Here's how the part is built. I have some questions about the finished solid (model axes, mm). Round coordinates to 2 decimals unless told otherwise and drop trailing zeros. Write each loop counter-clockwise with the first axis right and the second up, starting at its lowest first coordinate (ties: lowest second). Pieces come first, ordered by that corner, then holes. Notation, with made-up numbers: M 9,59.25 L 54,59.25 A19 cw 54,81.25 Z; hole C 63.25,-28 d7. An arc over 180 degrees is marked long. Use a Markdown table: item, result. Add a question column.
```python
from build123d import *

# Parameters (mm, degrees)
BOSS_EXTRUDE1_DEPTH = 152.4
SKETCH3_OUTSIDE_W   = 237.922
SKETCH3_OUTSIDE_H   = 226.36
CUT_EXTRUDE2_DEPTH  = 365.792952335
SHELL1_T            = -6.35
SKETCH8_W           = 266.062607669
SKETCH8_H           = 282.191647152
CUT_EXTRUDE6_DEPTH  = 300.618382774
CUT_EXTRUDE3_DEPTH  = 350.742043935
SKETCH5_OUTSIDE_W   = 351.444
SKETCH5_OUTSIDE_H   = 196.758
CUT_EXTRUDE4_DEPTH  = 296.012320666


with BuildPart() as part:
    # Sketch2 → Boss-Extrude1 (new body)
    with BuildSketch(Plane(origin=(0, 0, 0), x_dir=(1, 0, 0), z_dir=(0, 1, 0))):
        Polygon((-57.15, 0), (224.536, 0), (-24.357683353, -163.961583236), align=None)
    extrude(amount=BOSS_EXTRUDE1_DEPTH)

    # Sketch3 outside → Cut-Extrude2 (cut, through all)
    with BuildSketch(Plane(origin=(-63.5, 0, 0), x_dir=(0, 0, -1), z_dir=(1, 0, 0))):
        with Locations((-81.981, 76.2)):
            Rectangle(SKETCH3_OUTSIDE_W, SKETCH3_OUTSIDE_H)
        Polygon((0, 152.4), (-127, 107.95), (-217.714285714, 76.2), (-127, 44.45), (0, 0), align=None, mode=Mode.SUBTRACT)
    extrude(amount=CUT_EXTRUDE2_DEPTH, mode=Mode.SUBTRACT)

    # Shell1
    shell1_openings = [part.faces().sort_by_distance(p)[0] for p in [
        (83.693, 76.2, 0),
    ]]
    offset(amount=SHELL1_T, openings=shell1_openings, kind=Kind.INTERSECTION)

    # Sketch8 → Cut-Extrude6 (cut, through all)
    with BuildSketch(Plane.XY.offset(127)):
        with Locations((40.834882022, 90.229060284)):
            Rectangle(SKETCH8_W, SKETCH8_H)
    extrude(amount=CUT_EXTRUDE6_DEPTH, mode=Mode.SUBTRACT)

    # Sketch4 → Cut-Extrude3 (cut, through all)
    with BuildSketch(Plane(origin=(-63.5, 0, 0), x_dir=(0, 0, -1), z_dir=(1, 0, 0))):
        Polygon((0, 152.4), (0, 145.672295618), (-163.961583236, 88.285741485), (-163.961583236, 95.013445867), align=None)
        Polygon((-163.961583236, 64.114258515), (0, 6.727704382), (0, 0), (-163.961583236, 57.386554133), align=None)
    extrude(amount=CUT_EXTRUDE3_DEPTH, mode=Mode.SUBTRACT)


with BuildPart() as cut_extrude3_piece_1:
    # of the separate pieces the step leaves, piece 1, a body of its own (cut_extrude3_pieces)
    add(part.part.solids().sort_by_distance((224.536, 6.727704382, 0))[0])


with BuildPart() as cut_extrude3_piece_2:
    # of the separate pieces the step leaves, piece 2, a body of its own (cut_extrude3_pieces)
    add(part.part.solids().sort_by_distance((-31.75, 51.177704382, 127))[0])

    # Sketch5 outside → Cut-Extrude4 (cut, through all)
    with BuildSketch(Plane(origin=(0, 149.86, 0), x_dir=(1, 0, 0), z_dir=(0, 1, 0))):
        with Locations((83.693, -63.5)):
            Rectangle(SKETCH5_OUTSIDE_W, SKETCH5_OUTSIDE_H)
        Polygon((-20.197755363, -152.382449275), (-18.635799907, -160.192226553), (344.317071882, -160.192226553), (317.879717865, 72.864270331), (-35.136715197, 43.31663937), align=None, mode=Mode.SUBTRACT)
    extrude(amount=-CUT_EXTRUDE4_DEPTH, mode=Mode.SUBTRACT)


solid = cut_extrude3_piece_1.part
```
Item 1: Imagine slicing it at A-A on y = 67. List the corners of the cut face in (x, z) for me, plus the area to 3 significant figures.
Item 2: I need wall thicknesses on probe 1 along Z at (x, y) = (115.5, 94.5); probe 2 along X at (y, z) = (63, 108.5); probe 3 along X at (y, z) = (50.5, 105). Which ranges of each line are inside material? Lowest first, please. Write a range as from..to.
Item 3: For pin 1 Ø1 at (y, z) = (40, 50.5) entering from +X; pin 2 Ø1.5 at (y, z) = (121.5, 20) entering from -X; pin 3 Ø1 at (y, z) = (36, 66.5) entering from +X, each with a flat end and sliding along its axis, tell me the tip position at first contact or that it passes through.
Item 4: Imagine slicing it at B-B on z = 82. List the corners of the cut face in (x, y) for me.
The answers:
| question | item | result |
|---|---|---|
| 1 | outline | M 20.21,127 L 212.99,0 L 224.54,0 L 31.75,127 Z |
| 1 | area | 1,470 mm² |
| 2 | probe 1 | 64.22..71.83 |
| 2 | probe 2 | 48.29..59.83 |
| 2 | probe 3 | 53.6..65.15 |
| 3 | pin 1 | x = 148.64 |
| 3 | pin 2 | x = 181.49 |
| 3 | pin 3 | x = 124.35 |
| 4 | outline | M 88.52,35.43 L 100.06,35.43 L 100.06,116.97 L 88.52,116.97 Z |
